```python
from build123d import *

# Parameters (mm, degrees)
SKETCH_1_W          = 45
SKETCH_1_H          = 37
EXTRUDE_1_DEPTH     = 2
SKETCH_2_W          = 28
SKETCH_2_H          = 29
EXTRUDE_2_DEPTH     = 2
SKETCH_3_R          = 1.25
CUT_EXTRUDE_1_DEPTH = 2
SKETCH_4_W          = 8
SKETCH_4_H          = 18
EXTRUDE_3_DEPTH     = 6


with BuildPart() as part:
    # 草图1 → 凸台-拉伸1 (new body)
    with BuildSketch(Plane(origin=(0, 0, 0), x_dir=(1, 0, 0), z_dir=(0, 1, 0))):
        with Locations((22.5, 18.5)):
            Rectangle(SKETCH_1_W, SKETCH_1_H)
    extrude(amount=EXTRUDE_1_DEPTH)

    # 草图2 → 凸台-拉伸2 (add)
    with BuildSketch(Plane(origin=(0, 2, 0), x_dir=(1, 0, 0), z_dir=(0, 1, 0))):
        with Locations((22.5, 21.5)):
            Rectangle(SKETCH_2_W, SKETCH_2_H)
    extrude(amount=EXTRUDE_2_DEPTH)

    # 草图3 → 切除-拉伸1 (cut)
    with BuildSketch(Plane(origin=(0, 2, 0), x_dir=(1, 0, 0), z_dir=(0, 1, 0))):
        with Locations(Location((2.5, 35, 0), (0, 0, 270))):
            Circle(SKETCH_3_R)
        with Locations(Location((42.5, 35, 0), (0, 0, 90))):
            Circle(SKETCH_3_R)
        with Locations(Location((42.5, 2, 0), (0, 0, 270))):
            Circle(SKETCH_3_R)
        with Locations(Location((2.5, 2, 0), (0, 0, 90))):
            Circle(SKETCH_3_R)
    extrude(amount=-CUT_EXTRUDE_1_DEPTH, mode=Mode.SUBTRACT)

    # 草图4 → 凸台-拉伸3 (add)
    with BuildSketch(Plane.XZ):
        with Locations((41, -18.5)):
            Rectangle(SKETCH_4_W, SKETCH_4_H)
    extrude(amount=EXTRUDE_3_DEPTH)


solid = part.part
```
Geometry check sheet. Reference: the model listing, model coordinates, mm. A direction names the side the tool comes from. Give positions to 0.01 mm unless a question says otherwise; leave off trailing zeros. Loops run counter-clockwise (first coordinate to the right, second up) from the corner with the lowest first, then second, coordinate; pieces in that order, holes last. Notation, with made-up numbers: M 43,9 L 78,9 A21 ccw 78,22 Z; hole C -5.5,82 d9. An arc over 180 degrees is marked long. Write item = value, one per line. Start each with the question number.
1. Section check C-C, the plane z = -21.5. Enter the section's corners in (x, y).
2. Section check A-A, the plane x = 42.5. Enter the section's corners in (y, z), plus the area to 3 significant figures.
3. Go/stop test with flat-tipped pins: P1, Ø4, axis at x = 42.5, z = -35, coming from the +Y side; P2, Ø12, axis at x = 19, z = -31, coming from the -Y side; P3, Ø6, axis at y = -1, z = -29.5, coming from the +X side; P4, Ø3, axis at x = 40, y = -3.5, coming from the -Z side. Record where each tip stops, or that it passes through.
4. Section check B-B, the plane z = -35. Enter the section's corners in (x, y).
5. Draft check along X on faces 4 (the face through (8.5, 3, -21)), 5 (the face through (41.26, 1.01, -34.84)), 6 (the face through (43.74, 1.01, -2.16)), 7 (the face through (22, 2, -6)). Enter one of: +X half, -X half, draft (parallel to the pull), parting line (faces both ways), or undercut.
6. Section check D-D, the plane x = 19. Enter the section's corners in (y, z), plus the area to 3 significant figures.
7. Tool access check on faces 1 (the face through (37, -3, -19)), 2 (the face through (22, 3, -36)), 3 (the face through (41, -3, -9.5)). Record the directions out of +Z, -Z, +X, -X, +Y, -Y that give a thin tool (end or side, any length) a straight path to the whole face; none if there is none.
8. Thickness scan on probe 1 along X at (y, z) = (1.25, -35); probe 2 along Y at (x, z) = (25, -23); probe 3 along Y at (x, z) = (43.5, -8). Record the ranges inside material, lowest first.
Values follow:
q1.outline = M 0,0 L 37,0 L 37,-6 L 45,-6 L 45,2 L 36.5,2 L 36.5,4 L 8.5,4 L 8.5,2 L 0,2 Z
q2.outline = M -6,-27.5 L 0,-27.5 L 0,-33.75 L 2,-33.75 L 2,-3.25 L 0,-3.25 L 0,-9.5 L -6,-9.5 Z; M 0,-37 L 2,-37 L 2,-36.25 L 0,-36.25 Z; M 0,-0.75 L 2,-0.75 L 2,0 L 0,0 Z
q2.area = 172 mm^2
q3.P1 = 2
q3.P2 = 0
q3.P3 = 45
q3.P4 = -27.5
q4.outline = M 0,0 L 1.25,0 L 1.25,2 L 0,2 Z; M 3.75,0 L 41.25,0 L 41.25,2 L 36.5,2 L 36.5,4 L 8.5,4 L 8.5,2 L 3.75,2 Z; M 43.75,0 L 45,0 L 45,2 L 43.75,2 Z
q5.face_4 = -X half
q5.face_5 = undercut
q5.face_6 = undercut
q5.face_7 = draft
q6.outline = M 0,-37 L 2,-37 L 2,-36 L 4,-36 L 4,-7 L 2,-7 L 2,0 L 0,0 Z
q6.area = 132 mm^2
q7.face_1 = +Z, -Z, -X, -Y
q7.face_2 = -Z, +X, -X, +Y
q7.face_3 = +Z, +X, -X, -Y
q8.probe_1 = 0 to 1.25, 3.75 to 41.25, 43.75 to 45
q8.probe_2 = 0 to 4
q8.probe_3 = 0 to 2
